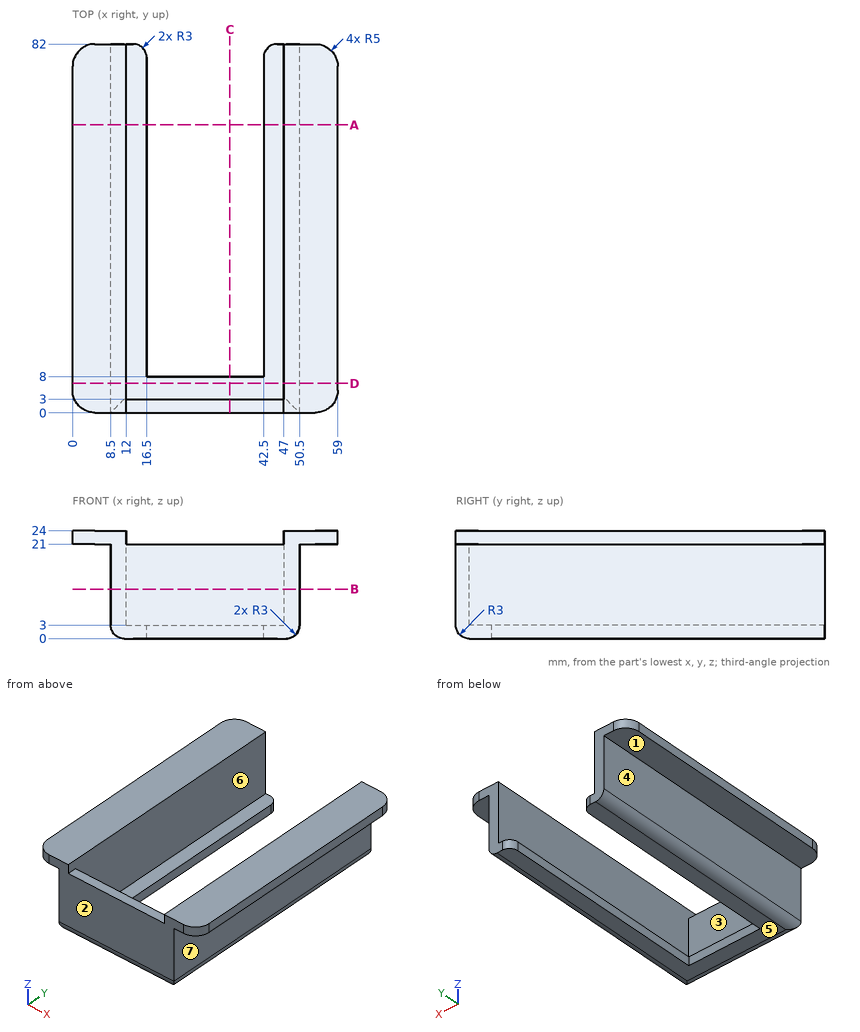
Answer from the drawing. Dimensions are ordinates in mm from the lowest x, y and z of the part. A direction names the side the tool comes from. Give positions to 0.01 mm unless a question says otherwise; leave off trailing zeros. Order: outer loops, then holes, each group sorted by start corner. A loop starts at its lowest first (then second) coordinate and runs counter-clockwise, first axis right, second up. Notation, with made-up numbers: (73.25, -40) - (126.25, -40) arc R21 cw to (126.25, -36) - close; hole circle Ø8 at (-14, 33.25). An arc over 180 degrees is marked (long way). One line per item, written item: value. Start each with the question number.
1) A cutting plane is placed at A-A on y = 64. Give the vertices of the cut face in (x, z).
2) A tool of negligible diameter and unlimited length cuts with its end or side. For the marked faces 1, 2 and 3, from which of +Z, -Z, +X, -X, +Y, -Y can it reach the whole face along a straight path? Write none if from no direction.
3) A cutting plane is placed at C-C on x = 35. Give the vertices of the cut face in (y, z), then the cut area to 3 significant figures.
4) Find the intervals of material crossed by L1, parallel to X at y = 28, z = 19.5; L2, parallel to X at y = 6.5, z = 21.75; L3, parallel to Y at x = 23.5, z = 19.5, in increasing order.
5) The mould has two halves that part along X. Classify the marked faces 4, 5, 6 and 7: released by +X, released by -X, zero draft, split by the parting line, or undercut.
6) A cutting plane is placed at B-B on z = 11. Give the vertices of the cut face in (x, y).
7) Given pin 1 Ø0.9 at (x, z) = (32, 2) entering from +Y; pin 2 Ø10 at (y, z) = (58, 6) entering from +X; pin 3 Ø4 at (x, y) = (55.5, 54.5) entering from -Z, each flat-ended and moving along its own axis, determine where each tip first touches the part or whether it passes through.
8) A cutting plane is placed at D-D on y = 6.5. Give the vertices of the cut face in (x, z), then the cut area to 3 significant figures.
Answer sheet:
1. outline: (0, 21) - (8.5, 21) - (8.5, 3) arc R3 ccw to (11.5, 0) - (16.5, 0) - (16.5, 3) - (12, 3) - (12, 24) - (0, 24) - close; (42.5, 0) - (47.5, 0) arc R3 ccw to (50.5, 3) - (50.5, 21) - (59, 21) - (59, 24) - (47, 24) - (47, 3) - (42.5, 3) - close
2. face 1: -Z, -X, +Y, -Y
2. face 2: +Z, -Z, +X, -X, -Y
2. face 3: +Z, +Y
3. outline: (0, 3) arc R3 ccw to (3, 0) - (8, 0) - (8, 3) - (3, 3) - (3, 21) - (0, 21) - close
3. area: 76.1 mm2
4. L1: x = 8.5 to 12, 47 to 50.5
4. L2: x = 0 to 12, 47 to 59
4. L3: y = 0 to 3
5. face 4: released by -X
5. face 5: zero draft
5. face 6: undercut
5. face 7: released by +X
6. outline: (8.5, 0) - (50.5, 0) - (50.5, 82) - (47, 82) - (47, 3) - (12, 3) - (12, 82) - (8.5, 82) - close
7. pin 1: stops at y = 8
7. pin 2: stops at x = 50.5
7. pin 3: stops at z = 21
8. outline: (0, 21) - (8.5, 21) - (8.5, 3) arc R3 ccw to (11.5, 0) - (47.5, 0) arc R3 ccw to (50.5, 3) - (50.5, 21) - (59, 21) - (59, 24) - (47, 24) - (47, 3) - (12, 3) - (12, 24) - (0, 24) - close
8. area: 320 mm2
